CAD build for the part. Positions are in the model's coordinates, mm. Face numbers are marked on the shaded views. A direction names the side the tool comes from. Give positions to 0.01 mm unless a question says otherwise; leave off trailing zeros. Order: outer loops, then holes, each group sorted by start corner. A loop starts at its lowest first (then second) coordinate and runs counter-clockwise, first axis right, second up. Notation, with made-up numbers: (32.5, -8) -> (85.5, -8) arc R25 ccw to (85.5, 19) -> close; hole circle Ø4 at (-38, 60). An arc over 180 degrees is marked (long way). Use one line per item in the form item = value. Start each with the question number.
1) Tool access for the marked faces 1 and 2: list every direction of +Z, -Z, +X, -X, +Y, -Y with a clear straight run to the whole face (end or side of a thin tool).
2) Cut at B-B, the plane y = 0.5. Give the cut face in (x, z).
3) Cut at C-C, the plane x = 24. Give the cut face in (y, z).
4) Drop a flat-ended pin along its axis: P1, Ø1.8, axis at x = 0, y = 31, coming from the -Z side. Give the stop position or say it passes through.
5) Cut at A-A, the plane z = 0.85. Give the cut face in (x, y).
6) Probe line 1 (Y direction, x = 0, z = 1.8); line 2 (X direction, y = -0.5, z = 2.95); line 3 (Y direction, x = 21, z = 2.6). List the from-to ranges inside material, lowest first.
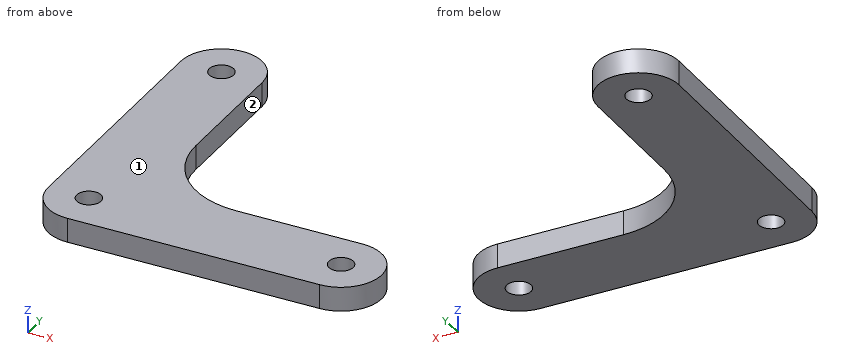
from build123d import *

# Parameters (mm, degrees)
SKETCH_R  = 1.5
PAD_DEPTH = 3
FILLET_R  = 10.5


with BuildPart() as part:
    # Sketch → Pad (new body)
    with BuildSketch(Plane.XY):
        with BuildLine():
            ThreePointArc((5, 31), (1.2e-05, 36), (-5, 31.000024))
            Line((-5, 0), (-5, 31.000024))
            ThreePointArc((-5, 0), (-3.535534, -3.535534), (0, -5))
            Line((31.000001, -5), (0, -5))
            ThreePointArc((31.000001, -5), (36, 0), (31, 5))
            Line((31, 5), (5, 5))
            Line((5, 31), (5, 5))
        make_face()
        Circle(SKETCH_R, mode=Mode.SUBTRACT)
        with Locations((0, 31)):
            Circle(SKETCH_R, mode=Mode.SUBTRACT)
        with Locations((31, 0)):
            Circle(SKETCH_R, mode=Mode.SUBTRACT)
    extrude(amount=PAD_DEPTH)

    # Fillet
    fillet_edges = [part.edges().sort_by_distance(p)[0] for p in [
        (5, 5, 1.5),
    ]]
    fillet(fillet_edges, radius=FILLET_R)


solid = part.part
Result:
q1.face_1 = +Z, +X, -X, +Y, -Y
q1.face_2 = +Z, -Z, +X, +Y
q2.outline = (-5, 0) -> (-1.41, 0) -> (-1.41, 3) -> (-5, 3) -> close; (1.41, 0) -> (29.59, 0) -> (29.59, 3) -> (1.41, 3) -> close; (32.41, 0) -> (35.97, 0) -> (35.97, 3) -> (32.41, 3) -> close
q3.outline = (-5, 0) -> (5, 0) -> (5, 3) -> (-5, 3) -> close
q4.P1 = through
q5.outline = (-5, 0) arc R5 ccw to (0, -5) -> (31, -5) arc R5 ccw to (31, 5) -> (15.5, 5) arc R10.5 cw to (5, 15.5) -> (5, 31) arc R5 ccw to (-5, 31) -> close; hole circle Ø3 at (0, 0); hole circle Ø3 at (0, 31); hole circle Ø3 at (31, 0)
q6.line_1 = -5 to -1.5, 1.5 to 29.5, 32.5 to 36
q6.line_2 = -4.97 to -1.41, 1.41 to 29.59, 32.41 to 35.97
q6.line_3 = -5 to 5
